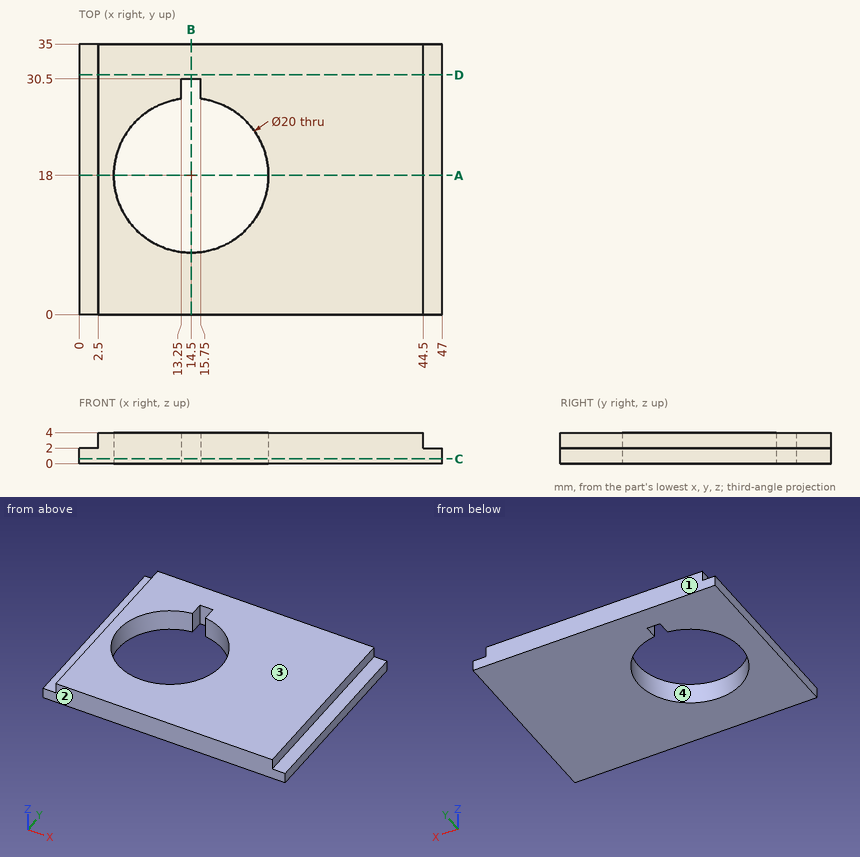
Here's the drawing with two shaded views (mm, measured from the low corner). I have some questions. Coordinates: 2 decimals unless noted, no trailing zeros. Write each loop counter-clockwise with the first axis right and the second up, starting at its lowest first coordinate (ties: lowest second). Pieces come first, ordered by that corner, then holes. Notation, with made-up numbers: (28.5, 44.5) - (39.5, 44.5) arc R17 ccw to (39.5, 50.5) - close; hole circle Ø7 at (25.25, -21). An arc over 180 degrees is marked (long way). Return JSON: item names as keys, results as strings.
Q1. If we section it at D-D (y = 31): Please give me the cut outline in (x, z), then the cut area to 3 significant figures.
Computed values:
{"outline": "(0, 0) - (47, 0) - (47, 2) - (44.5, 2) - (44.5, 4) - (2.5, 4) - (2.5, 2) - (0, 2) - close", "area": "178 mm2"}
Q2. If we section it at C-C (z = 0.6): Please give me the cut outline in (x, y).
Computed values:
{"outline": "(0, 0) - (47, 0) - (47, 35) - (0, 35) - close; hole (13.25, 27.92) arc R10 ccw (long way) to (15.75, 27.92) - (15.75, 30.5) - (13.25, 30.5) - close"}
Q3. If we section it at A-A (y = 18): Please give me the cut outline in (x, z).
Computed values:
{"outline": "(0, 0) - (4.5, 0) - (4.5, 4) - (2.5, 4) - (2.5, 2) - (0, 2) - close; (24.5, 0) - (47, 0) - (47, 2) - (44.5, 2) - (44.5, 4) - (24.5, 4) - close"}
Q4. I'm going to push flat-ended pins straight in: pin 1 Ø12 at (x, y) = (36, 29.5) entering from -Z; pin 2 Ø2 at (y, z) = (25, 3.5) entering from +X; pin 3 Ø18 at (x, y) = (14.5, 18) entering from +Z. Where does each tip first touch, or does it pass through?
Computed values:
{"pin 1": "stops at z = 0", "pin 2": "stops at x = 44.5", "pin 3": "passes through"}
Q5. Please list where these lines run through material, in increasing order: L1, parallel to X at y = 18, z = 1.8; L2, parallel to X at y = 29, z = 3.65; L3, parallel to Z at x = 45, y = 24. Write a range as from..to.
Computed values:
{"L1": "x = 0..4.5, 24.5..47", "L2": "x = 2.5..13.25, 15.75..44.5", "L3": "z = 0..2"}
Q6. Thinking about a two-plate mould opening in Y: for the marked faces 1, 2, 3 and 4, which applies, +Y half, -Y half, draft (parallel to the pull), parting line (faces both ways), or undercut?
Computed values:
{"face 1": "+Y half", "face 2": "-Y half", "face 3": "draft", "face 4": "undercut"}
Q7. If we section it at B-B (x = 14.5): Please give me the cut outline in (y, z), then the cut area to 3 significant figures.
Computed values:
{"outline": "(0, 0) - (8, 0) - (8, 4) - (0, 4) - close; (30.5, 0) - (35, 0) - (35, 4) - (30.5, 4) - close", "area": "50.0 mm2"}
